```python
from build123d import *

# Parameters (mm, degrees)
F0_W      = 12.9061160609
F0_H      = 30
F1_DEPTH  = 25
F2_DEPTH  = 10
F3_W      = 6.5
F3_H      = 10
F4_DEPTH  = 10
F5_W      = 6.5
F5_H      = 10
F6_DEPTH  = 10
F7_W      = 15
F7_H      = 30
F8_DEPTH  = 22.9061160609
F9_W      = 10
F9_H      = 10
F10_DEPTH = 6.5
F11_W     = 3
F11_H     = 5
F12_DEPTH = 10


with BuildPart() as f1:
    # F0 (on Front) → F1 (new body)
    with BuildSketch(Plane.XZ):
        with Locations((18.5469419695, 0)):
            Rectangle(F0_W, F0_H)
    extrude(amount=F1_DEPTH)



with BuildPart() as f1b:
    # F0 (on Front) → F1, piece 2 (new body)
    with BuildSketch(Plane.XZ):
        with Locations((-18.5469419695, 0)):
            Rectangle(F0_W, F0_H)
    extrude(amount=F1_DEPTH)


with BuildPart() as f1_1:
    add(f1.part)

    add(f1b.part)  # F2 merges F1b
    # F0 (on Front) → F2 (join)
    with BuildSketch(Plane.XZ):
        Polygon((25, 15), (25, 25), (-25, 25), (-25, 15), (-12.0938839391, 15), (-12.0938839391, -15), (-25, -15), (-25, -25), (25, -25), (25, -15), (12.0938839391, -15), (12.0938839391, 15), align=None)
    extrude(amount=F2_DEPTH)

    # F3 (on face) → F4 (join)
    with BuildSketch(Plane.YZ.offset(-12.0938839391)):
        with Locations((-21.75, 0)):
            Rectangle(F3_W, F3_H)
    extrude(amount=F4_DEPTH)

    # F5 (on face) → F6 (join)
    with BuildSketch(Plane(origin=(12.0938839391, 0, 0), x_dir=(0, -1, 0), z_dir=(-1, 0, 0))):
        with Locations((21.75, 0)):
            Rectangle(F5_W, F5_H)
    extrude(amount=F6_DEPTH)

    # F7 (on face) → F8 (cut, through all)
    with BuildSketch(Plane(origin=(-25, 0, 0), x_dir=(0, -1, 0), z_dir=(-1, 0, 0))):
        with Locations((17.5, 0)):
            Rectangle(F7_W, F7_H)
    extrude(amount=-F8_DEPTH, mode=Mode.SUBTRACT)

    # F9 (on face) → F10 (join)
    with BuildSketch(Plane.XZ.offset(25)):
        with Locations((7.0938839391, 0)):
            Rectangle(F9_W, F9_H)
    extrude(amount=F10_DEPTH)

    # F11 (on face) → F12 (cut)
    with BuildSketch(Plane.XZ.offset(10)):
        with Locations((-20, 7.5)):
            Rectangle(F11_W, F11_H)
    extrude(amount=-F12_DEPTH, mode=Mode.SUBTRACT)


solid = f1_1.part
```
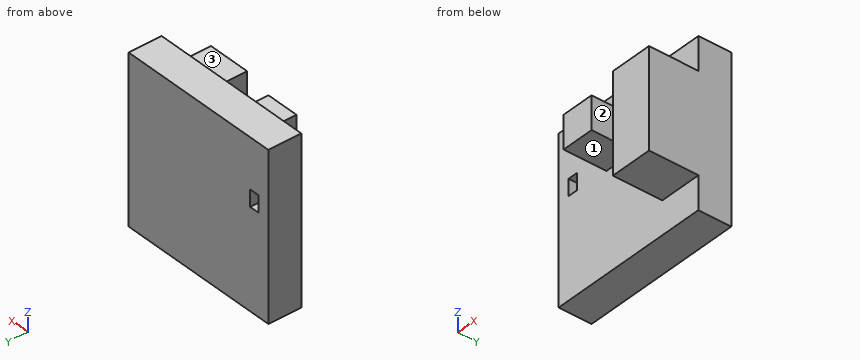
Here's how the part is built. I have some questions about the finished solid (model axes, mm). Face numbers are marked on the shaded views. A direction names the side the tool comes from. Coordinates: 2 decimals unless noted, no trailing zeros. Write each loop counter-clockwise with the first axis right and the second up, starting at its lowest first coordinate (ties: lowest second). Pieces come first, ordered by that corner, then holes. Notation, with made-up numbers: M -15,-4 L 6,-4 A21 cw 6,35 Z; hole C 30,31 d1. An arc over 180 degrees is marked long. Answer as CSV lines item,"result". Start each with the question number.
Q1. Suppose I cut it at D-D, the plane y = -15. List the corners of the cut face in (x, z) for me, then the cut area to 3 significant figures.
Q2. Suppose I cut it at C-C, the plane x = 19.5. List the corners of the cut face in (y, z) for me, then the cut area to 3 significant figures.
Q3. Suppose I cut it at A-A, the plane x = 6.5. List the corners of the cut face in (y, z) for me, then the cut area to 3 significant figures.
Q4. Suppose I cut it at B-B, the plane z = 9. List the corners of the cut face in (x, y) for me, then the cut area to 3 significant figures.
Q5. Will these pins go through, and if not, where does the flat tip stop? pin 1 Ø4 at (x, z) = (-3.5, -2.5) entering from -Y; pin 2 Ø14 at (x, y) = (16.5, -21) entering from +Z; pin 3 Ø12 at (y, z) = (-20.5, 2.5) entering from -X.
Q6. I need wall thicknesses on probe 1 along Y at (x, z) = (6, 4.5); probe 2 along Z at (x, y) = (-21, -5.5); probe 3 along X at (y, z) = (-11, 9.5). Which ranges of each line are inside material? Lowest first, please. Write a range as [from, to].
Q7. For the marked faces 1, 2 and 3, which set-ups out of +Z, -Z, +X, -X, +Y, -Y let a thin tool reach every point of the face, with its end or its side?
Entries:
1,outline,"M 12.09,-15 L 25,-15 L 25,15 L 12.09,15 Z"
1,area,"387 mm²"
2,outline,"M -25,-15 L -10,-15 L -10,-25 L 0,-25 L 0,25 L -10,25 L -10,15 L -25,15 Z"
2,area,"950 mm²"
3,outline,"M -31.5,-5 L -18.5,-5 L -18.5,5 L -31.5,5 Z; M -10,-25 L 0,-25 L 0,25 L -10,25 Z"
3,area,"630 mm²"
4,outline,"M -25,-10 L -21.5,-10 L -21.5,0 L -25,0 Z; M -18.5,-10 L 12.09,-10 L 12.09,-25 L 25,-25 L 25,0 L -18.5,0 Z"
4,area,"664 mm²"
5,pin 1,"stops at y = -10"
5,pin 2,"stops at z = 15"
5,pin 3,"stops at x = 2.09"
6,probe 1,"y = [-31.5, -18.5], [-10, 0]"
6,probe 2,"z = [-25, 5], [10, 25]"
6,probe 3,"x = [12.09, 25]"
7,face 1,"-Z, -X, -Y"
7,face 2,"+Z, -Z, +X, -Y"
7,face 3,"+Z, +X, -X, -Y"
